Could you check a few things on this model? Use its own coordinates, in mm. Face numbers are marked on the shaded views. Coordinates: 2 decimals unless noted, no trailing zeros. Order: outer loops, then holes, each group sorted by start corner. A loop starts at its lowest first (then second) coordinate and runs counter-clockwise, first axis right, second up. Notation, with made-up numbers: (9, -29) - (57, -29) arc R16 ccw to (57, -1) - close; hole circle Ø7 at (-11, 10.5). An arc over 180 degrees is marked (long way). Answer as CSV lines item,"result". Start each with the question number.
1. I want a section at C-C, the plane z = -4.5. List the corners of the cut face in (x, y) for me.
2. I want a section at B-B, the plane y = 2.6. List the corners of the cut face in (x, z) for me.
3. Thinking about a two-plate mould opening in X: for the marked faces 1, 2, 3 and 4, which applies, released by +X, released by -X, zero draft, split by the parting line, or undercut?
4. I want a section at D-D, the plane z = 10. List the corners of the cut face in (x, y) for me, and give its area (3 significant figures).
5. I want a section at A-A, the plane x = 0. List the corners of the cut face in (y, z) for me.
6. I need wall thicknesses on probe 1 along Z at (x, y) = (0, 2.7); probe 2 along Z at (x, y) = (1.5, 2); probe 3 along X at (y, z) = (0.2, -17). Which ranges of each line are inside material? Lowest first, please.
from build123d import *

# Parameters (mm, degrees)
BOSS_EXTRUDE1_DEPTH      = 20
BOSS_EXTRUDE1_DEPTH_BACK = 20


with BuildPart() as part:
    # Sketch1 → Boss-Extrude1 (new body, two sides)
    with BuildSketch(Plane.XY) as boss_extrude1_sk:
        with BuildLine():
            Line((-4.560050506, 0), (4.560050506, 0))
            ThreePointArc((4.560050506, 0), (5.206766179, 0.432121597), (5.055025253, 1.194974747))
            Line((5.055025253, 1.194974747), (2.455025253, 3.794974747))
            ThreePointArc((2.455025253, 3.794974747), (2.227928909, 3.946715673), (1.960050506, 4))
            Line((1.960050506, 4), (-1.960050506, 4))
            ThreePointArc((-1.960050506, 4), (-2.227928909, 3.946715673), (-2.455025253, 3.794974747))
            Line((-2.455025253, 3.794974747), (-5.055025253, 1.194974747))
            ThreePointArc((-5.055025253, 1.194974747), (-5.206766179, 0.432121597), (-4.560050506, 0))
        make_face()
    extrude(amount=BOSS_EXTRUDE1_DEPTH)
    extrude(boss_extrude1_sk.sketch, amount=-BOSS_EXTRUDE1_DEPTH_BACK)

    # Sketch2 → Cut-Revolve1 (revolve, cut)
    with BuildSketch(Plane(origin=(0, 0, 0), x_dir=(0, 0, -1), z_dir=(1, 0, 0))):
        Polygon((-10, 4), (-7.5, 4), (-7.933, 3.567), (-7.933, 0.433), (-7.5, 0), (-10, 0), align=None)
    revolve(axis=Axis((0, 0, 10), (0, 1, 0)), mode=Mode.SUBTRACT)

    # Sketch3 → Cut-Revolve2 (revolve, cut)
    with BuildSketch(Plane(origin=(0, 0, 0), x_dir=(0, 0, -1), z_dir=(1, 0, 0))):
        Polygon((10, 4), (12.5, 4), (12.067, 3.567), (12.067, 0.433), (12.5, 0), (10, 0), align=None)
    revolve(axis=Axis((0, 0, -10), (0, 1, 0)), mode=Mode.SUBTRACT)


solid = part.part
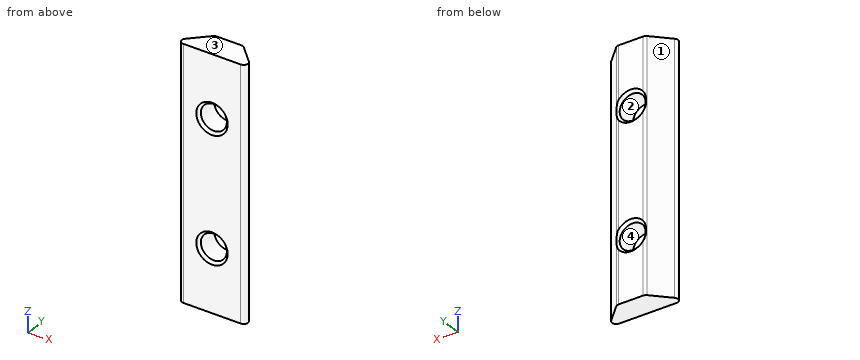
Solved:
1,outline,"(-5.06, 1.19) arc R0.7 ccw to (-4.56, 0) - (4.56, 0) arc R0.7 ccw to (5.06, 1.19) - (2.46, 3.79) arc R0.7 ccw to (1.96, 4) - (-1.96, 4) arc R0.7 ccw to (-2.46, 3.79) - close"
2,outline,"(-3.65, -20) - (3.65, -20) - (3.65, 20) - (-3.65, 20) - close; hole circle Ø4.13 at (0, -10); hole circle Ø4.13 at (0, 10)"
3,face 1,"released by -X"
3,face 2,"undercut"
3,face 3,"zero draft"
3,face 4,"undercut"
4,outline,"(-5.06, 1.19) arc R0.7 ccw to (-4.56, 0) - (-2.5, 0) - (-2.07, 0.43) - (-2.07, 3.57) - (-2.37, 3.87) arc R0.7 ccw to (-2.46, 3.79) - close; (2.07, 0.43) - (2.5, 0) - (4.56, 0) arc R0.7 ccw to (5.06, 1.19) - (2.46, 3.79) arc R0.7 ccw to (2.37, 3.87) - (2.07, 3.57) - close"
4,area,"15.9 mm2"
5,outline,"(0, -20) - (4, -20) - (4, -12.5) - (3.57, -12.07) - (0.43, -12.07) - (0, -12.5) - close; (0, -7.5) - (0.43, -7.93) - (3.57, -7.93) - (4, -7.5) - (4, 7.5) - (3.57, 7.93) - (0.43, 7.93) - (0, 7.5) - close; (0, 12.5) - (0.43, 12.07) - (3.57, 12.07) - (4, 12.5) - (4, 20) - (0, 20) - close"
6,probe 1,"z = -20 to -12.07, -7.93 to 7.93, 12.07 to 20"
6,probe 2,"z = -20 to -11.42, -8.58 to 8.58, 11.42 to 20"
6,probe 3,"x = -5.05 to 5.05"
